Design review of the part built by this model. Coordinates are the model's own, in mm. A direction names the side the tool comes from. Give positions to 0.01 mm unless a question says otherwise; leave off trailing zeros. Write each loop counter-clockwise with the first axis right and the second up, starting at its lowest first coordinate (ties: lowest second). Pieces come first, ordered by that corner, then holes. Notation, with made-up numbers: (30, 87) -> (81, 87) arc R16 cw to (81, 96) -> close; hole circle Ø8 at (28, 55.25). An arc over 180 degrees is marked (long way). Answer as a JSON object with one key per item and string values.
```python
from build123d import *

# Parameters (mm, degrees)
SKETCH1_R           = 2.9
BOSS_EXTRUDE1_DEPTH = 5.6
SKETCH2_R           = 17
CUT_EXTRUDE1_DEPTH  = 71.008603139


with BuildPart() as part:
    # Sketch1 → Boss-Extrude1 (new body)
    with BuildSketch(Plane.XY):
        with BuildLine():
            Line((-10, -4.142135624), (-10, -24))
            Line((-10, -24), (10, -24))
            Line((10, -24), (10, 4.142135624))
            Line((10, 4.142135624), (-10.026414893, 24.168550517))
            ThreePointArc((-10.026414893, 24.168550517), (-43.487067043, 43.487067043), (-24.168550517, 10.026414893))
            Line((-24.168550517, 10.026414893), (-10, -4.142135624))
        make_face()
        Circle(SKETCH1_R, mode=Mode.SUBTRACT)
    extrude(amount=BOSS_EXTRUDE1_DEPTH)

    # Sketch2 → Cut-Extrude1 (cut, through all)
    with BuildSketch(Plane.XY.offset(5.6)):
        with Locations((-29.344931419, 29.344931419)):
            Circle(SKETCH2_R)
    extrude(amount=-CUT_EXTRUDE1_DEPTH, mode=Mode.SUBTRACT)


solid = part.part
```
(1) For faces 4 (the flat face through (-10, -14, 3)), 5 (the cylindrical face through (-2.9, 0.1, 2.8)), list the 3-axis set-ups (+Z, -Z, +X, -X, +Y, -Y) from which the entire face can be reached by the end or side of a thin tool; tool diameter is ignored.
Here are the results:
{"face 4": "+Z, -Z, -X, -Y", "face 5": "+Z, -Z"}
(2) We need section D-D, the plane y = -15. State the section outline as (x, z) points.
Here are the results:
{"outline": "(-10, 0) -> (10, 0) -> (10, 5.6) -> (-10, 5.6) -> close"}
(3) Clearance check with flat-ended pins moving along their axes: pin 1 (2 mm diameter, centred on x = 1, y = -8.5, fed in from -Z); pin 2 (2 mm diameter, centred on x = 3, z = 3.5, fed in from +Y); pin 3 (3 mm diameter, centred on x = -21, z = 0.5, fed in from +Y); pin 4 (1.5 mm diameter, centred on x = 2, z = 3.5, fed in from +Y). State where each tip first meets the part, or that it passes through.
Here are the results:
{"pin 1": "stops at z = 0", "pin 2": "stops at y = 12.14", "pin 3": "stops at y = 48.14", "pin 4": "stops at y = 12.89"}
(4) We need section B-B, the plane z = 3.1. State the section outline as (x, y) points.
Here are the results:
{"outline": "(-24.17, 10.03) -> (-10, -4.14) -> (-10, -24) -> (10, -24) -> (10, 4.14) -> (-10.03, 24.17) arc R20 ccw (long way) to start; hole circle Ø34 at (-29.34, 29.34); hole circle Ø5.8 at (0, 0)"}
(5) The part is to be moulded in two halves that separate along Y. For faces 1 (the flat face through (-11, 7, 0)), 2 (the cylindrical face through (-31.56, 46.2, 2.84)), 3 (the flat face through (0, -24, 3)), say which applies: +Y half, -Y half, draft (parallel to the pull), parting line (faces both ways), or undercut.
Here are the results:
{"face 1": "draft", "face 2": "undercut", "face 3": "-Y half"}
(6) We need section A-A, the plane y = 41. State the section outline as (x, z) points, then the cut area to 3 significant figures.
Here are the results:
{"outline": "(-45.6, 0) -> (-41.72, 0) -> (-41.72, 5.6) -> (-45.6, 5.6) -> close; (-16.97, 0) -> (-13.09, 0) -> (-13.09, 5.6) -> (-16.97, 5.6) -> close", "area": "43.4 mm²"}
(7) For line 1 along Y through (x, z) = (-29, 2.4); line 2 along Y through (x, z) = (0, 1.45); line 3 along X through (y, z) = (-17, 3.25), list the stretches that pass through material, from the lowest coordinate up.
Here are the results:
{"line 1": "y = 9.35 to 12.35, 46.34 to 49.34", "line 2": "y = -24 to -2.9, 2.9 to 14.14", "line 3": "x = -10 to 10"}
(8) We need section C-C, the plane x = -34. State the section outline as (y, z) points, then the cut area to 3 significant figures.
Here are the results:
{"outline": "(9.89, 0) -> (12.99, 0) -> (12.99, 5.6) -> (9.89, 5.6) -> close; (45.7, 0) -> (48.8, 0) -> (48.8, 5.6) -> (45.7, 5.6) -> close", "area": "34.7 mm²"}
